Read the model definition and answer for the solid it produces. Units are mm, in the model's axes. Face numbers are marked on the shaded views. A direction names the side the tool comes from. Coordinates: 2 decimals unless noted, no trailing zeros. Loops run counter-clockwise (first coordinate to the right, second up) from the corner with the lowest first, then second, coordinate; pieces in that order, holes last.
Q1. Flat-ended cylindrical pins translate along their axes: P1, Ø4.5, axis at y = 94, z = -2.5, coming from the -X side; P2, Ø3, axis at x = 40, z = -11.5, coming from the +Y side; P3, Ø1.5, axis at x = -44, z = 20.5, coming from the -Y side. Find the tip coordinate at first contact, or state that the pin passes through.
Q2. Section C-C (z = 6) is taken. Give the vertices of the cut face in (x, y), then the cut area to 3 significant figures.
Q3. Section D-D (y = 33.5) is taken. Give the vertices of the cut face in (x, z), then the cut area to 3 significant figures.
Q4. Which of the six approach directions +Z, -Z, +X, -X, +Y, -Y give full straight-line access (tool end or side, diameter ignored) to the marked faces 4, 5, 6 and 7?
Q5. The mould has two halves that part along Y. Classify the marked faces 1, 2 and 3: pulls with the +Y half, pulls with the -Y half, needs draft (parallel to the pull), parting line crosses it, or undercut.
Q6. Section A-A (x = -21.5) is taken. Give the vertices of the cut face in (y, z), then the cut area to 3 significant figures.
Q7. Straight lines are drawn through the part: line 1 (X direction, y = 70, z = -13); line 2 (Y direction, x = -45, z = 12); line 3 (Z direction, x = 22, y = 22.5). For each, find the intervals that lie inside material, in ascending order.
Q8. Section B-B (y = 70) is taken. Give the vertices of the cut face in (x, z).
from build123d import *

# Parameters (mm, degrees)
SKETCH1_R           = 15
BOSS_EXTRUDE1_DEPTH = 27.5
CUT_EXTRUDE1_REACH  = 129.989
SKETCH2_W           = 55
SKETCH2_H           = 15
BOSS_EXTRUDE2_DEPTH = 35
CUT_EXTRUDE2_REACH  = 129.989
SKETCH5_W           = 15
SKETCH5_H           = 20
CUT_EXTRUDE3_REACH  = 129.989
SKETCH6_W           = 25
SKETCH6_H           = 15


with BuildPart() as part:
    # Sketch1 → Boss-Extrude1 (new, symmetric)
    with BuildSketch(Plane.XY):
        with BuildLine():
            Line((0, 0), (0, 100))
            Line((0, 100), (-45, 100))
            ThreePointArc((-45, 100), (-75, 70), (-45, 40))
            Line((-45, 40), (-20, 40))
            Line((-20, 40), (-20, 0))
            Line((-20, 0), (0, 0))
        make_face()
        with Locations((-45, 70)):
            Circle(SKETCH1_R, mode=Mode.SUBTRACT)
    extrude(amount=BOSS_EXTRUDE1_DEPTH, both=True)

    # Sketch2 → Cut-Extrude1 (cut, up to next)
    with BuildSketch(Plane(origin=(0, 100, 0), x_dir=(1, 0, 0), z_dir=(0, 1, 0)), mode=Mode.PRIVATE) as cut_extrude1_sk1:
        with Locations((-47.5, 0)):
            Rectangle(SKETCH2_W, SKETCH2_H)
    cut_extrude1_tool1 = extrude(cut_extrude1_sk1.sketch, amount=-CUT_EXTRUDE1_REACH, mode=Mode.PRIVATE) & part.part
    add(cut_extrude1_tool1.solids().sort_by_distance((-47.5, 100, 0))[0], mode=Mode.SUBTRACT)

    # Sketch4 → Boss-Extrude2 (add)
    with BuildSketch(Plane(origin=(0, 0, -27.5), x_dir=(-1, 0, 0), z_dir=(0, 0, -1))):
        with BuildLine():
            Line((-45, 0), (0, 0))
            Line((0, 0), (0, 60))
            ThreePointArc((0, 60), (-10.251262658, 35.251262658), (-35, 25))
            Line((-35, 25), (-45, 25))
            Line((-45, 25), (-45, 0))
        make_face()
    extrude(amount=-BOSS_EXTRUDE2_DEPTH)

    # Sketch5 → Cut-Extrude2 (cut, up to next)
    with BuildSketch(Plane(origin=(0, 0, 0), x_dir=(0, 0, -1), z_dir=(1, 0, 0)), mode=Mode.PRIVATE) as cut_extrude2_sk1:
        with Locations((0, 75)):
            Rectangle(SKETCH5_W, SKETCH5_H)
    cut_extrude2_tool1 = extrude(cut_extrude2_sk1.sketch, amount=-CUT_EXTRUDE2_REACH, mode=Mode.PRIVATE) & part.part
    add(cut_extrude2_tool1.solids().sort_by_distance((0, 75, 0))[0], mode=Mode.SUBTRACT)

    # Sketch6 → Cut-Extrude3 (cut, up to next)
    with BuildSketch(Plane.XZ, mode=Mode.PRIVATE) as cut_extrude3_sk1:
        with Locations((22.5, -10)):
            Rectangle(SKETCH6_W, SKETCH6_H)
    cut_extrude3_tool1 = extrude(cut_extrude3_sk1.sketch, amount=-CUT_EXTRUDE3_REACH, mode=Mode.PRIVATE) & part.part
    add(cut_extrude3_tool1.solids().sort_by_distance((22.5, 0, -10))[0], mode=Mode.SUBTRACT)


solid = part.part
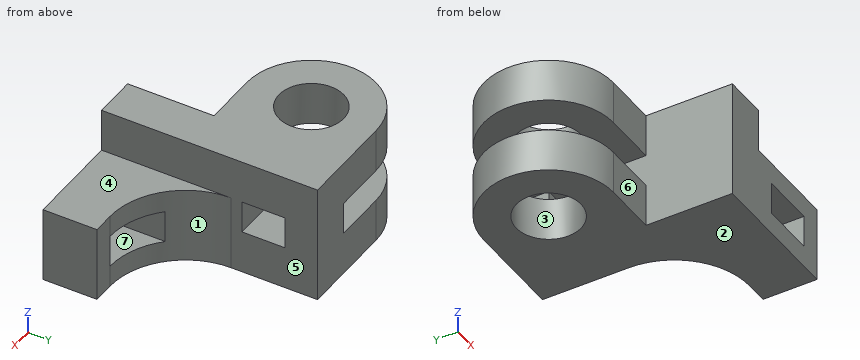
Numbers:
1. P1: stops at x = -20
1. P2: stops at y = 25
1. P3: stops at y = 40
2. outline: (-20, 0) - (45, 0) - (45, 25) - (35, 25) arc R35 cw to (0, 60) - (0, 65) - (-20, 65) - close; (-20, 85) - (0, 85) - (0, 100) - (-20, 100) - close
2. area: 2,990 mm2
3. outline: (-20, -27.5) - (12.14, -27.5) - (12.14, -17.5) - (10, -17.5) - (10, -2.5) - (12.14, -2.5) - (12.14, 7.5) - (0, 7.5) - (0, 27.5) - (-20, 27.5) - close
3. area: 1,490 mm2
4. face 4: +Z, +X, +Y, -Y
4. face 5: +Z, +X, +Y
4. face 6: +Z, -Z, -X, -Y
4. face 7: +Y, -Y
5. face 1: pulls with the +Y half
5. face 2: needs draft
5. face 3: undercut
6. outline: (40, -27.5) - (100, -27.5) - (100, -7.5) - (40, -7.5) - close; (40, 7.5) - (100, 7.5) - (100, 27.5) - (40, 27.5) - close
6. area: 2,400 mm2
7. line 1: x = -75 to -60, -30 to 0
7. line 2: y = 40 to 55, 85 to 100
7. line 3: z = -27.5 to -17.5, -2.5 to 7.5
8. outline: (-75, -27.5) - (-60, -27.5) - (-60, -7.5) - (-75, -7.5) - close; (-75, 7.5) - (-60, 7.5) - (-60, 27.5) - (-75, 27.5) - close; (-30, -27.5) - (0, -27.5) - (0, -7.5) - (-30, -7.5) - close; (-30, 7.5) - (0, 7.5) - (0, 27.5) - (-30, 27.5) - close
